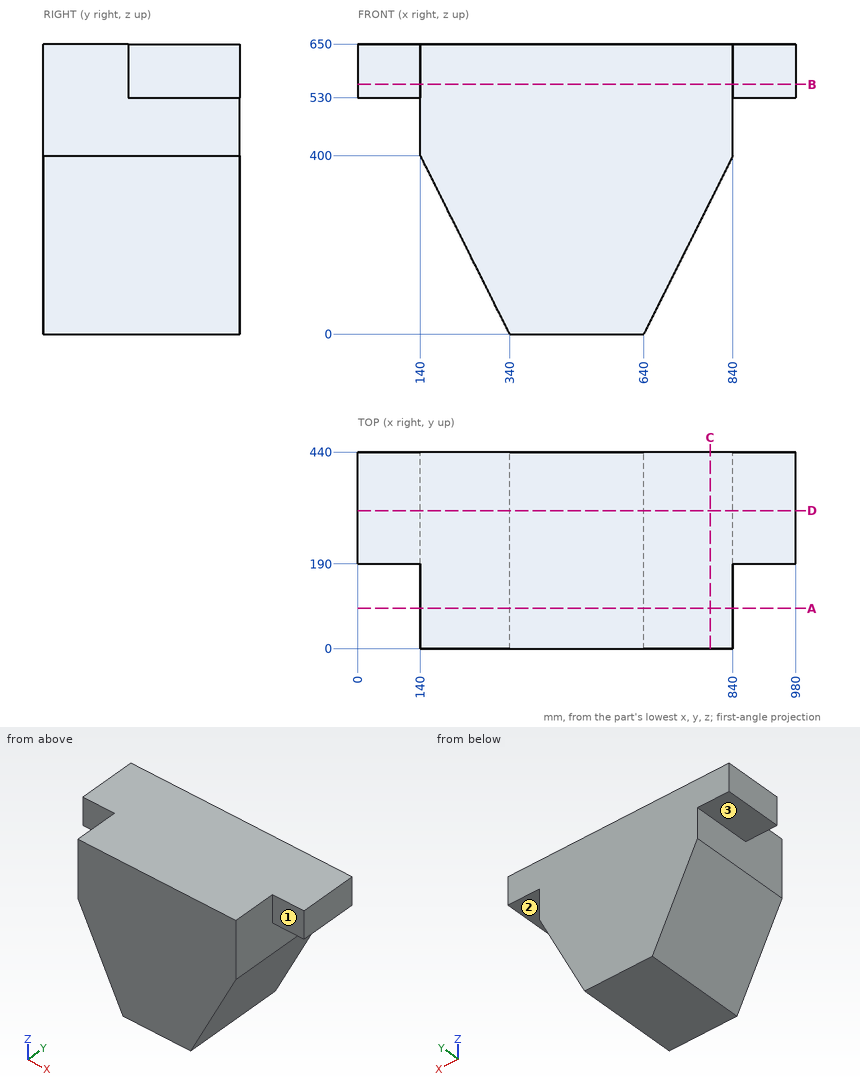
Check sheet for the drawn part. Datum: minimum x, y, z corner. Units: mm. A direction names the side the tool comes from. Round coordinates to 2 decimals unless told otherwise and drop trailing zeros. Order: outer loops, then holes, each group sorted by start corner. A loop starts at its lowest first (then second) coordinate and runs counter-clockwise, first axis right, second up. Notation, with made-up numbers: (72.25, 37.25) -> (90.25, 37.25) arc R17 cw to (90.25, 46.25) -> close; hole circle Ø3 at (57.25, 58). An arc over 180 degrees is marked (long way). Use CSV: the item, a comma, the result in double quotes.
(1) Cross-section at C-C (x = 789). Record the boundary of the cut face in (y, z).
Worked out:
outline,"(0, 298) -> (440, 298) -> (440, 650) -> (0, 650) -> close"
(2) Cross-section at D-D (y = 309). Record the boundary of the cut face in (x, z).
Worked out:
outline,"(0, 530) -> (140, 530) -> (140, 400) -> (340, 0) -> (640, 0) -> (840, 400) -> (840, 530) -> (980, 530) -> (980, 650) -> (0, 650) -> close"
(3) Tool access check on the marked faces 1, 2 and 3. Record the directions out of +Z, -Z, +X, -X, +Y, -Y that give a thin tool (end or side, any length) a straight path to the whole face; none if there is none.
Worked out:
face 1,"+Z, -Z, +X, -Y"
face 2,"-Z, +X, +Y, -Y"
face 3,"-Z, -X, +Y, -Y"
(4) Cross-section at A-A (y = 90). Record the boundary of the cut face in (x, z), and give its area (3 significant figures).
Worked out:
outline,"(140, 400) -> (340, 0) -> (640, 0) -> (840, 400) -> (840, 650) -> (140, 650) -> close"
area,"375,000 mm²"
(5) Material ranges on line 1 along Z through (x, y) = (854.5, 345.5); line 2 along X through (y, z) = (259.5, 447); line 3 along X through (y, z) = (112, 230), recorded low to high. Write a range as from..to.
Worked out:
line 1,"530..650"
line 2,"140..840"
line 3,"225..755"
(6) Cross-section at B-B (z = 559.5). Record the boundary of the cut face in (x, y), and give its area (3 significant figures).
Worked out:
outline,"(0, 190) -> (140, 190) -> (140, 0) -> (840, 0) -> (840, 190) -> (980, 190) -> (980, 440) -> (0, 440) -> close"
area,"378,000 mm²"
(7) Depth check by flat-ended pin: pin 1 (12 mm diameter, centred on y = 98.5, z = 358.5, fed in from +X); pin 2 (10 mm diameter, centred on y = 344, z = 275.5, fed in from -X); pin 3 (1 mm diameter, centred on y = 99, z = 366.5, fed in from -X). Enter the tip coordinate at first touch or a pass-through.
Worked out:
pin 1,"x = 822.25"
pin 2,"x = 199.75"
pin 3,"x = 156.5"
